Read the model definition and answer for the solid it produces. Units are mm, in the model's axes. A direction names the side the tool comes from. Round coordinates to 2 decimals unless told otherwise and drop trailing zeros. Order: outer loops, then holes, each group sorted by start corner. A loop starts at its lowest first (then second) coordinate and runs counter-clockwise, first axis right, second up. Notation, with made-up numbers: (-27, 68.5) - (1, 68.5) arc R14 ccw to (1, 80.5) - close; hole circle Ø4 at (9.25, 56.5). An arc over 180 degrees is marked (long way). One line per question, with ' | ' between items. Start each with the question number.
1) The mould has two halves that part along Z. Classify faces 1 (the flat face through (0, -80, -241.3)), 2 (the flat face through (0, 3, 292.1)), 3 (the flat face through (0, -222.25, 4)): pulls with the +Z half, pulls with the -Z half, needs draft (parallel to the pull), parting line crosses it, or undercut.
2) For faces 4 (the flat face through (0, 222.25, -178)), 5 (the flat face through (0, 192.881, -104)), 6 (the flat face through (0, 207, 63.5)), determine the directions among +Z, -Z, +X, -X, +Y, -Y from which every point of the face is accessible in a straight line to the end or side of a thin tool.
3) The part is cut by section C-C, the plane x = 0.75. Count the separate pieces of the cut face and the enclosed holes in it, plus the area to 3 significant figures.
4) Straight lines are drawn through the part: line 1 (Y direction, x = -2.5, z = 285.75) (3 decimals); line 2 (Y direction, x = 0.5, z = -215); line 3 (Y direction, x = 3.75, z = -120). For each, find the intervals that lie inside material, in ascending order. Write a range as from..to.
5) The part is cut by section B-B, the plane y = -79. Give the vertices of the cut face in (x, z).
6) The part is cut by section A-A, the plane z = 130. Give the vertices of the cut face in (x, y).
from build123d import *

# Parameters (mm, degrees)
SKETCH1_W                 = 12.7
SKETCH1_H                 = 444.5
EXTRUDE1_DEPTH            = 292.1
EXTRUDE1_DEPTH_BACK       = 292.1
CUT_EXTRUDE1_REACH        = 14.7
CUT_EXTRUDE2_REACH        = 14.7
SKETCH5_W                 = 127
SKETCH5_H                 = 43.65625
FILLET2_R                 = 6.35
M6X1_0_TAPPED_HOLE1_D     = 5
M6X1_0_TAPPED_HOLE1_DEPTH = 12.7
SKETCH11_W                = 292.1
SKETCH11_H                = 14.2875
CUT_EXTRUDE3_DEPTH        = 13.7
FILLET3_R                 = 3.175
CUT_EXTRUDE8_REACH        = 14.7
CUT_EXTRUDE7_DEPTH        = 1
CUT_EXTRUDE7_DEPTH_BACK   = 445.5
M6X1_0_TAPPED_HOLE2_D     = 5
M6X1_0_TAPPED_HOLE2_DEPTH = 12.7
M6_CLEARANCE_HOLE1_D      = 6.4
M6_CLEARANCE_HOLE1_DEPTH  = 12.7
M6X1_0_TAPPED_HOLE3_D     = 5
M6X1_0_TAPPED_HOLE3_DEPTH = 12.7
CUT_EXTRUDE9_DEPTH        = 13.7


with BuildPart() as part:
    # Sketch1 → Extrude1 (new body, two sides)
    with BuildSketch(Plane.XY) as extrude1_sk:
        Rectangle(SKETCH1_W, SKETCH1_H)
    extrude(amount=EXTRUDE1_DEPTH)
    extrude(extrude1_sk.sketch, amount=-EXTRUDE1_DEPTH_BACK)

    # Sketch4 → Cut-Extrude1 (cut, up to next)
    with BuildSketch(Plane(origin=(6.35, 0, 0), x_dir=(0, 0, -1), z_dir=(1, 0, 0)), mode=Mode.PRIVATE) as cut_extrude1_sk1:
        Polygon((203.2, 127.79375), (241.3, 127.79375), (241.3, 178.59375), (-241.3, 178.59375), (-241.3, 127.79375), (-203.2, 127.79375), (-203.2, -54.76875), (-241.3, -54.76875), (-241.3, -105.56875), (241.3, -105.56875), (241.3, -54.76875), (203.2, -54.76875), align=None)
    cut_extrude1_tool1 = extrude(cut_extrude1_sk1.sketch, amount=-CUT_EXTRUDE1_REACH, mode=Mode.PRIVATE) & part.part
    add(cut_extrude1_tool1.solids().sort_by_distance((6.35, 36.5125, 0))[0], mode=Mode.SUBTRACT)

    # Sketch5 → Cut-Extrude2 (cut, up to next)
    with BuildSketch(Plane(origin=(6.35, 0, 0), x_dir=(0, 0, -1), z_dir=(1, 0, 0)), mode=Mode.PRIVATE) as cut_extrude2_sk1:
        with Locations((0, 200.421875)):
            Rectangle(SKETCH5_W, SKETCH5_H)
    cut_extrude2_tool1 = extrude(cut_extrude2_sk1.sketch, amount=-CUT_EXTRUDE2_REACH, mode=Mode.PRIVATE) & part.part
    add(cut_extrude2_tool1.solids().sort_by_distance((6.35, 200.421875, 0))[0], mode=Mode.SUBTRACT)

    # Fillet2
    fillet2_edges = [part.edges().sort_by_distance(p)[0] for p in [
        (0, 127.79375, -203.2),
        (0, -54.76875, -203.2),
        (0, -54.76875, -241.3),
        (0, -105.56875, -241.3),
        (0, -105.56875, 241.3),
        (0, -54.76875, 241.3),
        (0, -54.76875, 203.2),
        (0, 127.79375, 203.2),
        (0, 127.79375, 241.3),
        (0, 178.59375, 241.3),
        (0, 178.59375, -241.3),
        (0, 127.79375, -241.3),
    ]]
    fillet(fillet2_edges, radius=FILLET2_R)

    # M6x1.0 Tapped Hole1
    with Locations(Plane(origin=(6.35, 0, 0), x_dir=(0, 0, -1), z_dir=(1, 0, 0))):
        with Locations((76.2, 204.7875), (-76.2, 204.7875), (101.6, -132.23875), (-101.6, -132.23875), (0, 204.7875)):
            Hole(M6X1_0_TAPPED_HOLE1_D / 2, depth=M6X1_0_TAPPED_HOLE1_DEPTH)

    # Sketch11 → Cut-Extrude3 (cut, through all)
    with BuildSketch(Plane(origin=(6.35, 0, 0), x_dir=(0, 0, -1), z_dir=(1, 0, 0))):
        with Locations((0, 185.7375)):
            Rectangle(SKETCH11_W, SKETCH11_H)
    extrude(amount=-CUT_EXTRUDE3_DEPTH, mode=Mode.SUBTRACT)

    # Fillet3
    fillet3_edges = [part.edges().sort_by_distance(p)[0] for p in [
        (0, 192.88125, 63.5),
        (0, 192.88125, -63.5),
        (0, 192.88125, 146.05),
        (0, 178.59375, -146.05),
        (0, 178.59375, 146.05),
        (0, 192.88125, -146.05),
        (0, 222.25, 63.5),
        (0, 222.25, -63.5),
    ]]
    fillet(fillet3_edges, radius=FILLET3_R)

    # Sketch19 → Cut-Extrude8 (cut, up to next)
    with BuildSketch(Plane(origin=(6.35, 0, 0), x_dir=(0, 0, -1), z_dir=(1, 0, 0)), mode=Mode.PRIVATE) as cut_extrude8_sk1:
        with BuildLine():
            Line((79.375, 207.9625), (79.375, 201.6125))
            ThreePointArc((79.375, 201.6125), (76.2, 198.4375), (73.025, 201.6125))
            Line((73.025, 201.6125), (73.025, 207.9625))
            ThreePointArc((73.025, 207.9625), (76.2, 211.1375), (79.375, 207.9625))
        make_face()
    cut_extrude8_tool1 = extrude(cut_extrude8_sk1.sketch, amount=-CUT_EXTRUDE8_REACH, mode=Mode.PRIVATE) & part.part
    add(cut_extrude8_tool1.solids().sort_by_distance((6.35, 204.7875, -76.2))[0], mode=Mode.SUBTRACT)
    # Sketch19 → Cut-Extrude8 (cut, up to next)
    with BuildSketch(Plane(origin=(6.35, 0, 0), x_dir=(0, 0, -1), z_dir=(1, 0, 0)), mode=Mode.PRIVATE) as cut_extrude8_sk2:
        with BuildLine():
            Line((-73.025, 207.9625), (-73.025, 201.6125))
            ThreePointArc((-73.025, 201.6125), (-76.2, 198.4375), (-79.375, 201.6125))
            Line((-79.375, 201.6125), (-79.375, 207.9625))
            ThreePointArc((-79.375, 207.9625), (-76.2, 211.1375), (-73.025, 207.9625))
        make_face()
    cut_extrude8_tool2 = extrude(cut_extrude8_sk2.sketch, amount=-CUT_EXTRUDE8_REACH, mode=Mode.PRIVATE) & part.part
    add(cut_extrude8_tool2.solids().sort_by_distance((6.35, 204.7875, 76.2))[0], mode=Mode.SUBTRACT)
    # Sketch19 → Cut-Extrude8 (cut, up to next)
    with BuildSketch(Plane(origin=(6.35, 0, 0), x_dir=(0, 0, -1), z_dir=(1, 0, 0)), mode=Mode.PRIVATE) as cut_extrude8_sk3:
        with BuildLine():
            Line((-98.425, -129.06375), (-98.425, -135.41375))
            ThreePointArc((-98.425, -135.41375), (-101.6, -138.58875), (-104.775, -135.41375))
            Line((-104.775, -135.41375), (-104.775, -129.06375))
            ThreePointArc((-104.775, -129.06375), (-101.6, -125.88875), (-98.425, -129.06375))
        make_face()
    cut_extrude8_tool3 = extrude(cut_extrude8_sk3.sketch, amount=-CUT_EXTRUDE8_REACH, mode=Mode.PRIVATE) & part.part
    add(cut_extrude8_tool3.solids().sort_by_distance((6.35, -132.23875, 101.6))[0], mode=Mode.SUBTRACT)
    # Sketch19 → Cut-Extrude8 (cut, up to next)
    with BuildSketch(Plane(origin=(6.35, 0, 0), x_dir=(0, 0, -1), z_dir=(1, 0, 0)), mode=Mode.PRIVATE) as cut_extrude8_sk4:
        with BuildLine():
            Line((104.775, -129.06375), (104.775, -135.41375))
            ThreePointArc((104.775, -135.41375), (101.6, -138.58875), (98.425, -135.41375))
            Line((98.425, -135.41375), (98.425, -129.06375))
            ThreePointArc((98.425, -129.06375), (101.6, -125.88875), (104.775, -129.06375))
        make_face()
    cut_extrude8_tool4 = extrude(cut_extrude8_sk4.sketch, amount=-CUT_EXTRUDE8_REACH, mode=Mode.PRIVATE) & part.part
    add(cut_extrude8_tool4.solids().sort_by_distance((6.35, -132.23875, -101.6))[0], mode=Mode.SUBTRACT)

    # Sketch18 → Cut-Extrude7 (cut, two sides)
    with BuildSketch(Plane.XZ.offset(222.25)) as cut_extrude7_sk:
        Polygon((6.35, 1.5875), (6.35, -1.5875), (4.7625, 0), align=None)
    extrude(amount=CUT_EXTRUDE7_DEPTH, mode=Mode.SUBTRACT)
    extrude(cut_extrude7_sk.sketch, amount=-CUT_EXTRUDE7_DEPTH_BACK, mode=Mode.SUBTRACT)

    # M6x1.0 Tapped Hole2
    with Locations(Plane(origin=(6.35, 0, 0), x_dir=(0, 0, -1), z_dir=(1, 0, 0))):
        with Locations((79.375, -191.29375), (-79.375, -191.29375), (250.825, -149.225), (250.825, 193.675), (-250.825, 193.675), (-250.825, -149.225)):
            Hole(M6X1_0_TAPPED_HOLE2_D / 2, depth=M6X1_0_TAPPED_HOLE2_DEPTH)

    # M6 Clearance Hole1
    with Locations(Plane(origin=(6.35, 0, 0), x_dir=(0, 0, -1), z_dir=(1, 0, 0))):
        with Locations((-285.75, -196.85), (-285.75, -66.675), (-285.75, 193.675), (-285.75, 63.5), (285.75, 193.675), (285.75, 63.5), (285.75, -66.675), (285.75, -196.85)):
            Hole(M6_CLEARANCE_HOLE1_D / 2, depth=M6_CLEARANCE_HOLE1_DEPTH)

    # M6x1.0 Tapped Hole3
    with Locations(Plane(origin=(6.35, 55.5625, 214.3125), x_dir=(0, 1, 0), z_dir=(1, 0, 0))):
        with Locations((0, 0), (-38.1, 0), (0, -428.625), (-38.1, -428.625)):
            Hole(M6X1_0_TAPPED_HOLE3_D / 2, depth=M6X1_0_TAPPED_HOLE3_DEPTH)

    # Sketch28 → Cut-Extrude9 (cut, through all)
    with BuildSketch(Plane(origin=(6.35, 0, 0), x_dir=(0, 0, -1), z_dir=(1, 0, 0))):
        with BuildLine():
            Line((-217.4875, 20.6375), (-211.1375, 20.6375))
            ThreePointArc((-211.1375, 20.6375), (-207.9625, 17.4625), (-211.1375, 14.2875))
            Line((-211.1375, 14.2875), (-217.4875, 14.2875))
            ThreePointArc((-217.4875, 14.2875), (-220.6625, 17.4625), (-217.4875, 20.6375))
        make_face()
        with BuildLine():
            Line((-217.4875, 58.7375), (-211.1375, 58.7375))
            ThreePointArc((-211.1375, 58.7375), (-207.9625, 55.5625), (-211.1375, 52.3875))
            Line((-211.1375, 52.3875), (-217.4875, 52.3875))
            ThreePointArc((-217.4875, 52.3875), (-220.6625, 55.5625), (-217.4875, 58.7375))
        make_face()
        with BuildLine():
            Line((-73.025, 201.6125), (-73.025, 207.9625))
            ThreePointArc((-73.025, 207.9625), (-76.2, 211.1375), (-79.375, 207.9625))
            Line((-79.375, 207.9625), (-79.375, 201.6125))
            ThreePointArc((-79.375, 201.6125), (-76.2, 198.4375), (-73.025, 201.6125))
        make_face()
        with BuildLine():
            Line((79.375, 201.6125), (79.375, 207.9625))
            ThreePointArc((79.375, 207.9625), (76.2, 211.1375), (73.025, 207.9625))
            Line((73.025, 207.9625), (73.025, 201.6125))
            ThreePointArc((73.025, 201.6125), (76.2, 198.4375), (79.375, 201.6125))
        make_face()
        with BuildLine():
            Line((104.775, -135.41375), (104.775, -129.06375))
            ThreePointArc((104.775, -129.06375), (101.6, -125.88875), (98.425, -129.06375))
            Line((98.425, -129.06375), (98.425, -135.41375))
            ThreePointArc((98.425, -135.41375), (101.6, -138.58875), (104.775, -135.41375))
        make_face()
        with BuildLine():
            Line((-98.425, -135.41375), (-98.425, -129.06375))
            ThreePointArc((-98.425, -129.06375), (-101.6, -125.88875), (-104.775, -129.06375))
            Line((-104.775, -129.06375), (-104.775, -135.41375))
            ThreePointArc((-104.775, -135.41375), (-101.6, -138.58875), (-98.425, -135.41375))
        make_face()
        with BuildLine():
            Line((211.1375, 58.7375), (217.4875, 58.7375))
            ThreePointArc((217.4875, 58.7375), (220.6625, 55.5625), (217.4875, 52.3875))
            Line((217.4875, 52.3875), (211.1375, 52.3875))
            ThreePointArc((211.1375, 52.3875), (207.9625, 55.5625), (211.1375, 58.7375))
        make_face()
        with BuildLine():
            Line((211.1375, 20.6375), (217.4875, 20.6375))
            ThreePointArc((217.4875, 20.6375), (220.6625, 17.4625), (217.4875, 14.2875))
            Line((217.4875, 14.2875), (211.1375, 14.2875))
            ThreePointArc((211.1375, 14.2875), (207.9625, 17.4625), (211.1375, 20.6375))
        make_face()
    extrude(amount=-CUT_EXTRUDE9_DEPTH, mode=Mode.SUBTRACT)


solid = part.part
Values:
1) face 1: undercut | face 2: pulls with the +Z half | face 3: needs draft
2) face 4: +Z, -Z, +X, -X, +Y | face 5: +X, -X | face 6: +X, -X, +Y
3) separate pieces: 1 | enclosed holes: 22 | area: 128,000 mm^2
4) line 1: y = -222.25..-200.05, -193.65..-69.875, -63.475..60.3, 66.7..190.475, 196.875..222.25 | line 2: y = -222.25..-105.57, -54.77..14.29, 20.64..52.39, 58.74..127.79, 178.59..222.25 | line 3: y = -222.25..-105.57, 192.88..222.25
5) outline: (-6.35, -292.1) - (6.35, -292.1) - (6.35, -241.3) - (-6.35, -241.3) - close; (-6.35, 241.3) - (6.35, 241.3) - (6.35, 292.1) - (-6.35, 292.1) - close
6) outline: (-6.35, -222.25) - (6.35, -222.25) - (6.35, -105.57) - (-6.35, -105.57) - close; (-6.35, 192.88) - (6.35, 192.88) - (6.35, 222.25) - (-6.35, 222.25) - close
